Source: CAD feature listing. Evaluate the final solid. Frame: model axes, mm. Give positions to 0.01 mm unless a question says otherwise; leave off trailing zeros. Loops run counter-clockwise (first coordinate to the right, second up) from the corner with the lowest first, then second, coordinate; pieces in that order, holes last. Notation, with made-up numbers: M 25.5,27.5 L 48.5,27.5 A22 ccw 48.5,60.5 Z; hole C 59,67.5 d7. An arc over 180 degrees is marked long. Put each result on its own line as item: value.
from build123d import *

# Parameters (mm, degrees)
SKETCH1_R           = 65
SKETCH1_R_2         = 40
BOSS_EXTRUDE1_DEPTH = 15
SKETCH2_R           = 3
CUT_EXTRUDE1_DEPTH  = 94.139680051
CIRPATTERN1_COUNT   = 6


with BuildPart() as part:
    # Sketch1 → Boss-Extrude1 (new body)
    with BuildSketch(Plane(origin=(0, 0, 0), x_dir=(1, 0, 0), z_dir=(0, 1, 0))):
        with Locations(Location((0, 0, 0), (0, 0, 270))):
            Circle(SKETCH1_R)
        with Locations(Location((0, 0, 0), (0, 0, 270))):
            Circle(SKETCH1_R_2, mode=Mode.SUBTRACT)
    extrude(amount=BOSS_EXTRUDE1_DEPTH)

    # Sketch2 → Cut-Extrude1 (cut, through all)
    with BuildSketch(Plane(origin=(0, 0, 0), x_dir=(0, 0, -1), z_dir=(1, 0, 0))):
        with Locations((0, 7.5)):
            Circle(SKETCH2_R)
    cut_extrude1 = extrude(amount=-CUT_EXTRUDE1_DEPTH, mode=Mode.SUBTRACT)

    # CirPattern1: Cut-Extrude1 ×6 about axis
    cirpattern1_axis = Axis((0, 15, 0), (0, 1, 0))
    for i in range(1, CIRPATTERN1_COUNT):
        add(cut_extrude1.rotate(cirpattern1_axis, i * 360 / CIRPATTERN1_COUNT), mode=Mode.SUBTRACT)


solid = part.part
1. Section query B-B (x = 0). Output: boundary loops of the cut face in (y, z), plus the area to 3 significant figures.
Found:
outline: M 0,-65 L 15,-65 L 15,-40 L 0,-40 Z; M 0,40 L 15,40 L 15,65 L 0,65 Z
area: 750 mm^2
2. Contact query for flat-ended pins moving along their axis: P1, Ø5, axis at y = 8, z = 3, coming from the +X side; P2, Ø1, axis at y = 5, z = -31.5, coming from the -X side; P3, Ø1.5, axis at x = 41.5, y = 9, coming from the -Z side. Output: stop coordinate, or through.
Found:
P1: x = 64.98
P2: x = -57.13
P3: z = -50.64
3. Section query C-C (y = 7.5). Output: boundary loops of the cut face in (x, z).
Found:
outline: M -64.93,-3 A65 ccw -35.06,-54.73 L -22.54,-33.04 A40 cw -39.89,-3 Z; M -64.93,3 L -39.89,3 A40 cw -22.54,33.04 L -35.06,54.73 A65 ccw Z; M -29.87,-57.73 A65 ccw 29.87,-57.73 L 17.35,-36.04 A40 cw -17.35,-36.04 Z; M -29.87,57.73 L -17.35,36.04 A40 cw 17.35,36.04 L 29.87,57.73 A65 ccw Z; M 22.54,-33.04 L 35.06,-54.73 A65 ccw 64.93,-3 L 39.89,-3 A40 cw Z; M 22.54,33.04 A40 cw 39.89,3 L 64.93,3 A65 ccw 35.06,54.73 Z
4. Material intervals for line 1 (Y direction, x = -45.75, z = 0); line 2 (Z direction, x = -25.5, y = 6.25); line 3 (Z direction, x = 49.25, y = 7.5), sorted ascending. Write a range as from..to.
Found:
line 1: 0..4.5, 10.5..15
line 2: -59.79..-49.62, -38.71..-30.82, 30.82..38.71, 49.62..59.79
line 3: -42.42..-3, 3..42.42
5. Section query A-A (z = 0). Output: boundary loops of the cut face in (x, y), plus the area to 3 significant figures.
Found:
outline: M -65,0 L -40,0 L -40,4.5 L -65,4.5 Z; M -65,10.5 L -40,10.5 L -40,15 L -65,15 Z; M 40,0 L 65,0 L 65,4.5 L 40,4.5 Z; M 40,10.5 L 65,10.5 L 65,15 L 40,15 Z
area: 450 mm^2
6. Section query D-D (z = -20). Output: boundary loops of the cut face in (x, y).
Found:
outline: M -61.85,0 L -34.64,0 L -34.64,15 L -61.85,15 Z; M 34.64,0 L 61.85,0 L 61.85,15 L 34.64,15 Z
7. Draft query along X for faces 1 (the flat face through (30, 0, 28)), 2 (the cylindrical face through (-39.05, 7.4, -8.67)), 3 (the cylindrical face through (19.52, 7.4, 62)). Return one class per face: pulls with the +X half, pulls with the -X half, needs draft (parallel to the pull), parting line crosses it, or undercut.
Found:
face 1: needs draft
face 2: undercut
face 3: parting line crosses it
